Work out the finished part from the listing and answer in its coordinate system (mm). A direction names the side the tool comes from. Give positions to 0.01 mm unless a question says otherwise; leave off trailing zeros. Write each loop counter-clockwise with the first axis right and the second up, starting at its lowest first coordinate (ties: lowest second). Pieces come first, ordered by that corner, then holes. Notation, with made-up numbers: (36, 35.5) -> (65, 35.5) arc R7 ccw to (65, 44.5) -> close; hole circle Ø8 at (78.25, -1). An arc over 180 degrees is marked (long way). Write item = value, one per line. Start each with the question number.
from build123d import *

# Parameters (mm, degrees)
ESQUISSE1_R             = 10.5
BOSS_EXTRU_1_DEPTH      = 25
ENL_V_MAT_EXTRU_1_DEPTH = 35
ENL_V_MAT_EXTRU_2_DEPTH = 50
ENL_V_MAT_EXTRU_3_DEPTH = 15
ESQUISSE1_4_R           = 6.5
ENL_V_MAT_EXTRU_4_DEPTH = 26
ESQUISSE1_5_R           = 10
ENL_V_MAT_EXTRU_5_DEPTH = 12


with BuildPart() as part:
    # Esquisse1 → Boss.-Extru.1 (new body)
    with BuildSketch(Plane.XY):
        with BuildLine():
            Line((600, -25), (0, -25))
            ThreePointArc((0, -25), (-25, 0), (0, 25))
            Line((0, 25), (600, 25))
            ThreePointArc((600, 25), (625, 0), (600, -25))
        make_face()
        Circle(ESQUISSE1_R, mode=Mode.SUBTRACT)
        with BuildLine():
            Line((560, 10.5), (600, 10.5))
            ThreePointArc((600, 10.5), (610.5, 0), (600, -10.5))
            Line((600, -10.5), (560, -10.5))
            ThreePointArc((560, -10.5), (549.5, 0), (560, 10.5))
        make_face(mode=Mode.SUBTRACT)
    extrude(amount=BOSS_EXTRU_1_DEPTH)

    # Esquisse2 → Enl_v. mat.-Extru.1 (cut)
    with BuildSketch(Plane(origin=(0, 25, 0), x_dir=(1, 0, 0), z_dir=(0, 1, 0))):
        Polygon((510, 0), (500, 0), (500, -5), (495, -5), (495, -10), (515, -10), (515, -5), (510, -5), align=None)
    extrude(amount=-ENL_V_MAT_EXTRU_1_DEPTH, mode=Mode.SUBTRACT)

    # Esquisse3 → Enl_v. mat.-Extru.2 (cut)
    with BuildSketch(Plane(origin=(0, 25, 0), x_dir=(1, 0, 0), z_dir=(0, 1, 0))):
        Polygon((19.49708464, 0), (19.49708464, -5), (14.49708464, -5), (14.49708464, -10), (34.49708464, -10), (34.49708464, -5.357949986), (29.49708464, -5.357949986), (29.49708464, 0), align=None)
    extrude(amount=-ENL_V_MAT_EXTRU_2_DEPTH, mode=Mode.SUBTRACT)

    # Esquisse1_3 → Enl_v. mat.-Extru.3 (cut)
    with BuildSketch(Plane.XY):
        Polygon((290, -25), (310, -25), (310, -20), (317.5, -20), (317.5, -15), (282.5, -15), (282.5, -20), (290, -20), align=None)
        Polygon((45, -25), (55, -25), (55, -20), (62.5, -20), (62.5, -15), (45, -15), align=None)
        Polygon((545, -25), (555, -25), (555, -15), (537.5, -15), (537.5, -20), (545, -20), align=None)
    extrude(amount=ENL_V_MAT_EXTRU_3_DEPTH, mode=Mode.SUBTRACT)

    # Esquisse1_4 → Enl_v. mat.-Extru.4 (cut, through all)
    with BuildSketch(Plane.XY):
        with Locations((300, 0)):
            Circle(ESQUISSE1_4_R)
        with Locations((450, 0)):
            Circle(ESQUISSE1_4_R)
        with Locations((150, 0)):
            Circle(ESQUISSE1_4_R)
    extrude(amount=ENL_V_MAT_EXTRU_4_DEPTH, mode=Mode.SUBTRACT)

    # Esquisse1_5 → Enl_v. mat.-Extru.5 (cut)
    with BuildSketch(Plane.XY):
        with Locations((300, 0)):
            Circle(ESQUISSE1_5_R)
        with Locations((450, 0)):
            Circle(ESQUISSE1_5_R)
        with Locations((150, 0)):
            Circle(ESQUISSE1_5_R)
    extrude(amount=ENL_V_MAT_EXTRU_5_DEPTH, mode=Mode.SUBTRACT)


solid = part.part
(1) A cutting plane is placed at B-B, the plane x = 150. Write down the section's boundary in (y, z), then the cut area to 3 significant figures.
(2) Find the intervals of material crossed by line 1 along Y through (x, z) = (300, 18.75); line 2 along X through (y, z) = (14.5, 4); line 3 along X through (y, z) = (6, 14.5), in increasing order.
(3) For faces 4 (the cylindrical face through (290, 0, 6)), 5 (the flat face through (45, -20, 7)), 6 (the flat face through (304, -25, 18)), 7 (the flat face through (505, 8, 10)), 8 (the flat face through (580, -10.5, 12)), determine the directions among +Z, -Z, +X, -X, +Y, -Y from which every point of the face is accessible in a straight line to the end or side of a thin tool.
(4) Determine the mould class of faces 1 (the cylindrical face through (624.994, 0.55, 12.325)), 2 (the flat face through (-2, 11, 0)), 3 (the flat face through (52, -19, 15)) for opening direction X: pulls with the +X half, pulls with the -X half, needs draft (parallel to the pull), parting line crosses it, or undercut.
(5) A cutting plane is placed at A-A, the plane x = 300. Write down the section's boundary in (y, z), then the cut area to 3 significant figures.
(6) Each of these flat-tipped pins is pushed along its axis until it touches: pin 1 (4 mm diameter, centred on y = -17.5, z = 6, fed in from +X); pin 2 (1.5 mm diameter, centred on y = -8, z = 1.5, fed in from +X); pin 3 (2.5 mm diameter, centred on y = -17.5, z = 10, fed in from +X). Where does it stop, or does it pass through?
Results list:
q1.outline = (-25, 0) -> (-10, 0) -> (-10, 12) -> (-6.5, 12) -> (-6.5, 25) -> (-25, 25) -> close; (6.5, 12) -> (10, 12) -> (10, 0) -> (25, 0) -> (25, 25) -> (6.5, 25) -> close
q1.area = 841 mm²
q2.line_1 = -25 to -6.5, 6.5 to 25
q2.line_2 = -20.37 to 19.5, 29.5 to 500, 510 to 620.37
q2.line_3 = -24.27 to -8.62, 8.62 to 147.5, 152.5 to 297.5, 302.5 to 447.5, 452.5 to 551.38, 608.62 to 624.27
q3.face_4 = -Z
q3.face_5 = -Z, -Y
q3.face_6 = +Z, -Z, +X, -X, -Y
q3.face_7 = +Y
q3.face_8 = +Z, -Z
q4.face_1 = pulls with the +X half
q4.face_2 = needs draft
q4.face_3 = undercut
q5.outline = (-25, 15) -> (-15, 15) -> (-15, 0) -> (-10, 0) -> (-10, 12) -> (-6.5, 12) -> (-6.5, 25) -> (-25, 25) -> close; (6.5, 12) -> (10, 12) -> (10, 0) -> (25, 0) -> (25, 25) -> (6.5, 25) -> close
q5.area = 691 mm²
q6.pin_1 = 619.62
q6.pin_2 = 623.93
q6.pin_3 = 619
